from build123d import *

# Parameters (mm, degrees)
BOSS_EXTRUDE1_DEPTH     = 25
SKETCH2_R               = 11
CUT_EXTRUDE1_DEPTH      = 26
CUT_EXTRUDE1_DEPTH_BACK = 26
SKETCH3_R               = 8
CUT_EXTRUDE2_DEPTH      = 35
SKETCH4_R               = 8
CUT_EXTRUDE3_DEPTH      = 30


with BuildPart() as part:
    # Sketch1 → Boss-Extrude1 (new body, symmetric)
    with BuildSketch(Plane.XY):
        Polygon((350, 232.421392473), (-350, 232.421392473), (-350, -67.578607527), (-65, -67.578607527), (-55, -57.578607527), (-55, 81.421392473), (55, 81.421392473), (55, -57.578607527), (65, -67.578607527), (350, -67.578607527), align=None)
    extrude(amount=BOSS_EXTRUDE1_DEPTH, both=True)

    # Sketch2 → Cut-Extrude1 (cut, two sides)
    with BuildSketch(Plane.XY) as cut_extrude1_sk:
        with Locations((0, 172.421392473)):
            Circle(SKETCH2_R)
    extrude(amount=CUT_EXTRUDE1_DEPTH, mode=Mode.SUBTRACT)
    extrude(cut_extrude1_sk.sketch, amount=-CUT_EXTRUDE1_DEPTH_BACK, mode=Mode.SUBTRACT)

    # Sketch3 → Cut-Extrude2 (cut)
    with BuildSketch(Plane(origin=(0, 232.421392473, 0), x_dir=(1, 0, 0), z_dir=(0, 1, 0))):
        Circle(SKETCH3_R)
    extrude(amount=-CUT_EXTRUDE2_DEPTH, mode=Mode.SUBTRACT)

    # Sketch4 → Cut-Extrude3 (cut)
    with BuildSketch(Plane.XZ.offset(67.578607527)):
        with Locations((-80, 0)):
            Circle(SKETCH4_R)
        with Locations((80, 0)):
            Circle(SKETCH4_R)
    extrude(amount=-CUT_EXTRUDE3_DEPTH, mode=Mode.SUBTRACT)


solid = part.part
Work out the finished part from the listing and answer in its coordinate system (mm). A direction names the side the tool comes from. Coordinates: 2 decimals unless noted, no trailing zeros. Loops run counter-clockwise (first coordinate to the right, second up) from the corner with the lowest first, then second, coordinate; pieces in that order, holes last. Notation, with made-up numbers: M 84.25,43.5 L 122.25,43.5 A11 cw 122.25,60.5 Z; hole C -6,11.5 d2. An arc over 180 degrees is marked long. Answer in a Markdown table with one row per item. Add a question column.
1. Consider L1, parallel to X at y = 218, z = -1; L2, parallel to Z at x = 80, y = -47.25; L3, parallel to X at y = 76.5, z = -3.5. Determine where each line is inside the solid, lowest interval first.
2. Find section B-B, the plane x = 0. Write down the section's boundary in (y, z).
3. The mould has two halves that part along Z. Classify faces 1 (the flat face through (-209, -67.579, 0)), 2 (the flat face through (80, -37.579, 0)), 3 (the flat face through (-5, 85, 25)): pulls with the +Z half, pulls with the -Z half, needs draft (parallel to the pull), parting line crosses it, or undercut.
4. Find section A-A, the plane y = -45. Write down the section's boundary in (x, z), then the cut area to 3 significant figures.
5. Find section C-C, the plane y = -9.5. Write down the section's boundary in (x, z), then the cut area to 3 significant figures.
6. Find section D-D, the plane z = 0. Write down the section's boundary in (x, y).
7. A tool of negligible diameter and unlimited length cuts with its end or side. For faces 4 (the cylindrical face through (-86.349, -52.789, -4.868)), 5 (the cylindrical face through (-1.73, 215.17, 7.81)), 6 (the flat face through (-55, 11, 0)), from which of +Z, -Z, +X, -X, +Y, -Y can it reach the whole face along a straight path? Write none if from no direction.
8. Flat-ended cylindrical pins translate along their axes: P1, Ø5, axis at x = 2.5, z = 1.5, coming from the +Y side; P2, Ø14.5, axis at x = 80, z = 0, coming from the -Y side; P3, Ø17.5, axis at x = 0, y = 172.42, coming from the -Z side; P4, Ø1, axis at x = -3, z = 4.5, coming from the -Y side. Find the tip coordinate at first contact, or state that the pin passes through.
Reported:
| question | item | result |
|---|---|---|
| 1 | L1 | x = -350 to -7.94, 7.94 to 350 |
| 1 | L2 | z = -25 to -8, 8 to 25 |
| 1 | L3 | x = -350 to -55, 55 to 350 |
| 2 | outline | M 81.42,-25 L 161.42,-25 L 161.42,25 L 81.42,25 Z; M 183.42,-25 L 232.42,-25 L 232.42,-8 L 197.42,-8 L 197.42,8 L 232.42,8 L 232.42,25 L 183.42,25 Z |
| 3 | face 1 | needs draft |
| 3 | face 2 | undercut |
| 3 | face 3 | pulls with the +Z half |
| 4 | outline | M -350,-25 L -55,-25 L -55,25 L -350,25 Z; M 55,-25 L 350,-25 L 350,25 L 55,25 Z; hole C -80,0 d16; hole C 80,0 d16 |
| 4 | area | 29,100 mm^2 |
| 5 | outline | M -350,-25 L -55,-25 L -55,25 L -350,25 Z; M 55,-25 L 350,-25 L 350,25 L 55,25 Z |
| 5 | area | 29,500 mm^2 |
| 6 | outline | M -350,-67.58 L -88,-67.58 L -88,-37.58 L -72,-37.58 L -72,-67.58 L -65,-67.58 L -55,-57.58 L -55,81.42 L 55,81.42 L 55,-57.58 L 65,-67.58 L 72,-67.58 L 72,-37.58 L 88,-37.58 L 88,-67.58 L 350,-67.58 L 350,232.42 L 8,232.42 L 8,197.42 L -8,197.42 L -8,232.42 L -350,232.42 Z; hole C 0,172.42 d22 |
| 7 | face 4 | -Y |
| 7 | face 5 | +Y |
| 7 | face 6 | +Z, -Z, -Y |
| 8 | P1 | stops at y = 197.42 |
| 8 | P2 | stops at y = -37.58 |
| 8 | P3 | passes through |
| 8 | P4 | stops at y = 81.42 |
